Verification items for the finished model (mm, model axes). Face numbers are marked on the shaded views. A direction names the side the tool comes from. Give positions to 0.01 mm unless a question says otherwise; leave off trailing zeros. Loops run counter-clockwise (first coordinate to the right, second up) from the corner with the lowest first, then second, coordinate; pieces in that order, holes last. Notation, with made-up numbers: M -38.5,59 L -31.5,59 A24 ccw -31.5,72 Z; hole C 13,74 d2. An arc over 180 degrees is marked long. Use a Markdown table: item, result.
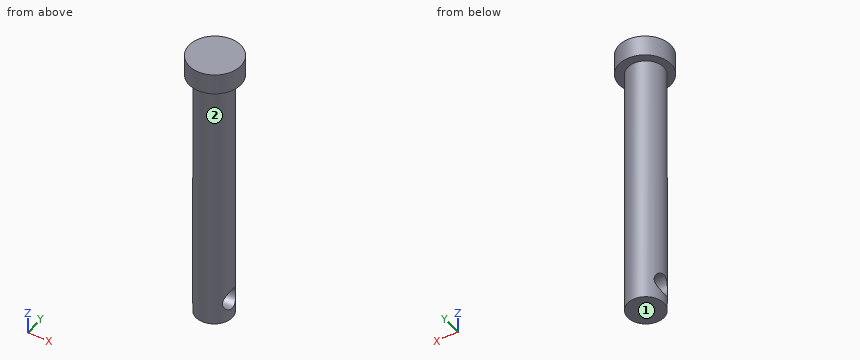
from build123d import *

# Parameters (mm, degrees)
SKETCH1_W               = 125
SKETCH1_H               = 8.75
BOSS_EXTRUDE1_START     = 62.5
BOSS_EXTRUDE1_OUTLINE_R = 12.5
BOSS_EXTRUDE1_DEPTH     = 10
CUT_EXTRUDE1_DEPTH      = 75.705524807
CUT_EXTRUDE1_DEPTH_BACK = 75.705524807
SKETCH2_R               = 5


# Read off the part's stored shape, not the designer's step: Boss-Extrude1
with BuildPart() as part:
    # Sketch1 → Revolve1 (revolve)
    with BuildSketch(Plane(origin=(0, 0, 0), x_dir=(0, 0, -1), z_dir=(1, 0, 0)), mode=Mode.PRIVATE) as revolve1_sk:
        with Locations((0, 4.375)):
            Rectangle(SKETCH1_W, SKETCH1_H)
    revolve(revolve1_sk.sketch.rotate(Axis((0, 0, 0), (0, 0, -1)), 90), axis=Axis((0, 0, 0), (0, 0, -1)))

    # Boss-Extrude1 outline → Boss-Extrude1 (add)
    with BuildSketch(Plane.XY.offset(BOSS_EXTRUDE1_START)):
        with Locations((0.232114028, 0.249851338)):
            Circle(BOSS_EXTRUDE1_OUTLINE_R)
    extrude(amount=BOSS_EXTRUDE1_DEPTH)

    # Sketch2 → Cut-Extrude1 (cut, two sides: drawn at the far end of the back side and taken through both)
    with BuildSketch(Plane(origin=(0, 0, 0), x_dir=(0, 0, -1), z_dir=(1, 0, 0)).offset(-CUT_EXTRUDE1_DEPTH_BACK)):
        with Locations((52.5, 0)):
            Circle(SKETCH2_R)
    extrude(amount=CUT_EXTRUDE1_DEPTH + CUT_EXTRUDE1_DEPTH_BACK, mode=Mode.SUBTRACT)


solid = part.part
(1) Cross-section at B-B on z = -52.5. Record the cut outline in (x, y), then the cut area to 3 significant figures.
Results below:
| item | result |
|---|---|
| outline | M -7.18,-5 A8.75 ccw 7.18,-5 Z; M -7.18,5 L 7.18,5 A8.75 ccw Z |
| area | 75.6 mm^2 |
(2) Gauge pin test, flat ends, axial feed: P1, Ø10, axis at x = 4.5, z = -2, coming from the +Y side; P2, Ø1.5, axis at x = 2.5, z = 48.5, coming from the -Y side; P3, Ø4, axis at y = 3.5, z = 1, coming from the +X side. Record the tip position at first contact, or that the pin passes through.
Results below:
| item | result |
|---|---|
| P1 | y = 8.75 |
| P2 | y = -8.57 |
| P3 | x = 8.62 |
(3) Cross-section at A-A on x = 0.25. Record the cut outline in (y, z), then the cut area to 3 significant figures.
Results below:
| item | result |
|---|---|
| outline | M -12.25,62.5 L -8.75,62.5 L -8.75,-62.5 L 8.75,-62.5 L 8.75,62.5 L 12.75,62.5 L 12.75,72.5 L -12.25,72.5 Z; hole C 0,-52.5 d10 |
| area | 2,360 mm^2 |
(4) Cross-section at D-D on z = 14.5. Record the cut outline in (x, y), then the cut area to 3 significant figures.
Results below:
| item | result |
|---|---|
| outline | C 0,0 d17.5 |
| area | 241 mm^2 |
(5) Set-up check for the marked faces 1 and 2: record each of +Z, -Z, +X, -X, +Y, -Y from which the full face is reachable in a straight line by a thin tool's end or side.
Results below:
| item | result |
|---|---|
| face 1 | -Z, +X, -X, +Y, -Y |
| face 2 | -Z |
(6) Material ranges on line 1 (Z direction, x = -0.5, y = 0); line 2 (Y direction, x = -0.5, z = 8.5); line 3 (Y direction, x = -3, z = -52.5), recorded low to high.
Results below:
| item | result |
|---|---|
| line 1 | -62.5 to -57.5, -47.5 to 72.5 |
| line 2 | -8.74 to 8.74 |
| line 3 | -8.22 to -5, 5 to 8.22 |
(7) Cross-section at C-C on x = 6.75. Record the cut outline in (y, z), then the cut area to 3 significant figures.
Results below:
| item | result |
|---|---|
| outline | M -10.42,62.5 L -5.57,62.5 L -5.57,-62.5 L 5.57,-62.5 L 5.57,62.5 L 10.92,62.5 L 10.92,72.5 L -10.42,72.5 Z; hole C 0,-52.5 d10 |
| area | 1,530 mm^2 |
